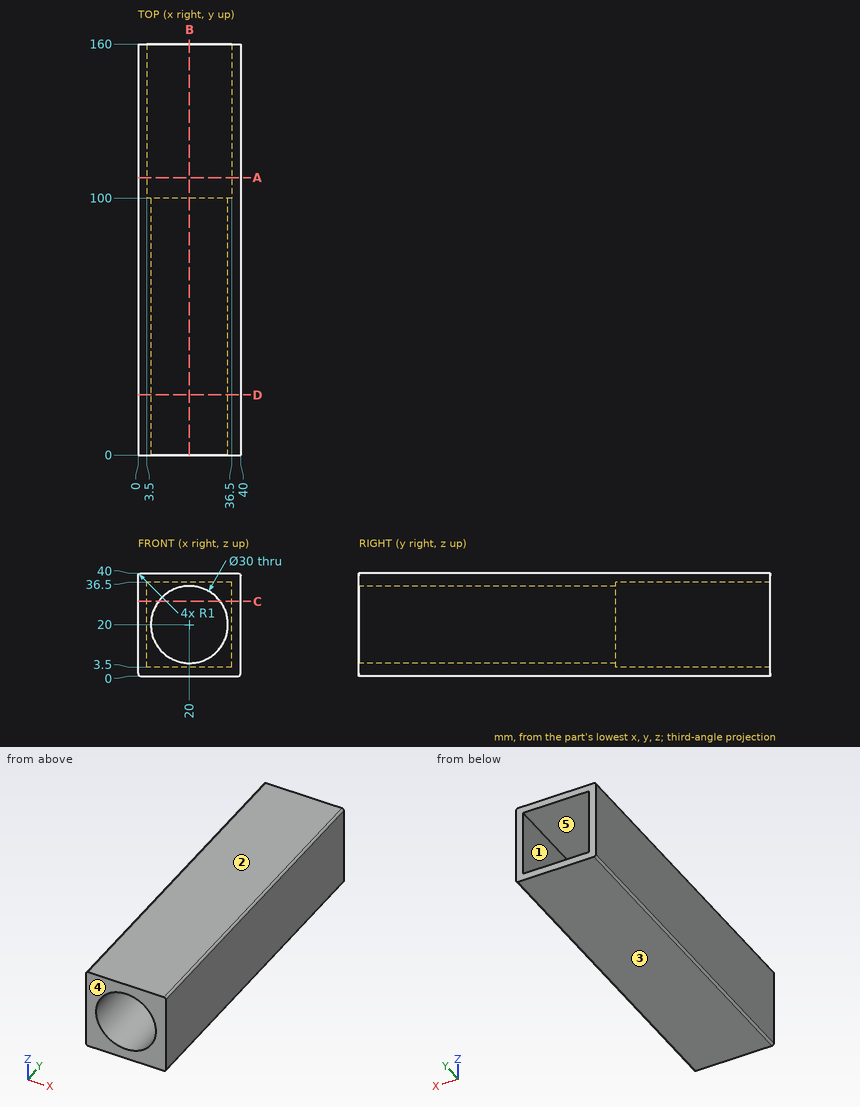
Could you check a few things on this drawing? It's one solid part, dimensions in mm from its lowest x, y, z. A direction names the side the tool comes from. Give positions to 0.01 mm unless a question says otherwise; leave off trailing zeros. Order: outer loops, then holes, each group sorted by start corner. A loop starts at its lowest first (then second) coordinate and runs counter-clockwise, first axis right, second up. Notation, with made-up numbers: (44.5, -27) - (58.5, -27) arc R22 cw to (58.5, -1) - close; hole circle Ø3 at (53.5, 56). An arc over 180 degrees is marked (long way). One line per item, written item: value. Start each with the question number.
1. Imagine slicing it at C-C on z = 29. List the corners of the cut face in (x, y) for me, plus the area to 3 significant figures.
2. Imagine slicing it at D-D on y = 23.5. List the corners of the cut face in (x, z) for me.
3. If I drill on probe 1 along Z at (x, y) = (17, 108.5); probe 2 along Z at (x, y) = (20, 40), over which ranges is the centre line in solid material (lowest first)?
4. Thinking about a two-plate mould opening in Z: for the marked faces 1, 2 and 3, which applies, +Z half, -Z half, draft (parallel to the pull), parting line (faces both ways), or undercut?
5. For the marked faces 4 and 5, which set-ups out of +Z, -Z, +X, -X, +Y, -Y let a thin tool reach every point of the face, with its end or its side?
6. For P1, Ø2, axis at y = 55.5, z = 26, coming from the -X side; P2, Ø4, axis at x = 17, z = 31.5, coming from the -Y side; P3, Ø2, axis at x = 32.5, z = 30, coming from the +Y side, each with a flat end and sliding along its axis, tell me the tip position at first contact or that it passes through.
7. Imagine slicing it at A-A on y = 108. List the corners of the cut face in (x, z) for me.
8. Imagine slicing it at B-B on x = 20. List the corners of the cut face in (y, z) for me, plus the area to 3 significant figures.
Values:
1. outline: (0, 0) - (8, 0) - (8, 100) - (3.5, 100) - (3.5, 160) - (0, 160) - close; (32, 0) - (40, 0) - (40, 160) - (36.5, 160) - (36.5, 100) - (32, 100) - close
1. area: 2,020 mm²
2. outline: (0, 1) arc R1 ccw to (1, 0) - (39, 0) arc R1 ccw to (40, 1) - (40, 39) arc R1 ccw to (39, 40) - (1, 40) arc R1 ccw to (0, 39) - close; hole circle Ø30 at (20, 20)
3. probe 1: 0 to 3.5, 36.5 to 40
3. probe 2: 0 to 5, 35 to 40
4. face 1: undercut
4. face 2: +Z half
4. face 3: -Z half
5. face 4: +Z, -Z, +X, -X, -Y
5. face 5: +Y
6. P1: x = 0
6. P2: through
6. P3: y = 100
7. outline: (0, 1) arc R1 ccw to (1, 0) - (39, 0) arc R1 ccw to (40, 1) - (40, 39) arc R1 ccw to (39, 40) - (1, 40) arc R1 ccw to (0, 39) - close; hole (3.5, 3.5) - (36.5, 3.5) - (36.5, 36.5) - (3.5, 36.5) - close
8. outline: (0, 0) - (160, 0) - (160, 3.5) - (100, 3.5) - (100, 5) - (0, 5) - close; (0, 35) - (100, 35) - (100, 36.5) - (160, 36.5) - (160, 40) - (0, 40) - close
8. area: 1,420 mm²
